```python
from build123d import *

# Parameters (mm, degrees)
F0_R     = 6.35
F1_DEPTH = 3.175
F2_R     = 6.35
F4_DEPTH = 3.175
F5_COUNT = 4
F6_COUNT = 4


with BuildPart() as f1:
    # F0 (on Top) → F1 (new body)
    with BuildSketch(Plane.XY):
        with BuildLine():
            Line((4.7625, -143.2460284405), (4.7625, -9.1539715595))
            ThreePointArc((4.7625, -9.1539715595), (0, 10.31875), (-4.7625, -9.1539715595))
            Line((-4.7625, -9.1539715595), (-4.7625, -143.2460284405))
            ThreePointArc((-4.7625, -143.2460284405), (0, -162.71875), (4.7625, -143.2460284405))
        make_face()
        with Locations((0, -152.4)):
            Circle(F0_R, mode=Mode.SUBTRACT)
        Circle(F0_R, mode=Mode.SUBTRACT)
    extrude(amount=F1_DEPTH)

    # F2
    f2_edges = [f1.edges().sort_by_distance(p)[0] for p in [
        (4.7625, -9.153972, 1.5875),
        (-4.7625, -9.153972, 1.5875),
        (-4.7625, -143.246028, 1.5875),
        (4.7625, -143.246028, 1.5875),
    ]]
    fillet(f2_edges, radius=F2_R)

    # F3 (on face) → F4 (cut, through all)
    with BuildSketch(Plane.XY.offset(3.175)):
        with BuildLine():
            ThreePointArc((-5.8666350314, -154.8300397955), (-6.35, -152.4), (-5.8666350314, -149.9699602045))
            Line((-5.8666350314, -149.9699602045), (-6.5999644104, -149.66620523))
            ThreePointArc((-6.5999644104, -149.66620523), (-7.14375, -152.4), (-6.5999644104, -155.13379477))
            Line((-6.5999644104, -155.13379477), (-5.8666350314, -154.8300397955))
        make_face()
        with BuildLine():
            ThreePointArc((-5.8666350314, -2.4300397955), (-6.35, 0), (-5.8666350314, 2.4300397955))
            Line((-5.8666350314, 2.4300397955), (-6.5999644104, 2.73379477))
            ThreePointArc((-6.5999644104, 2.73379477), (-7.14375, 0), (-6.5999644104, -2.73379477))
            Line((-6.5999644104, -2.73379477), (-5.8666350314, -2.4300397955))
        make_face()
    f4 = extrude(amount=-F4_DEPTH, mode=Mode.SUBTRACT)

    # F5: F4 ×4 about axis
    f5_axis = Axis((0, -152.4, 3.175), (0, 0, 1))
    for i in range(1, F5_COUNT):
        add(f4.solids().sort_by_distance((-6.2333, -154.981917, 1.5875))[0].rotate(f5_axis, i * 360 / F5_COUNT), mode=Mode.SUBTRACT)

    # F6: F4 ×4 about axis
    f6_axis = Axis((0, 0, 3.175), (0, 0, 1))
    for i in range(1, F6_COUNT):
        add(f4.solids().sort_by_distance((-6.2333, 2.581917, 1.5875))[0].rotate(f6_axis, i * 360 / F6_COUNT), mode=Mode.SUBTRACT)


solid = f1.part
```
The listing builds one solid part. Answer for the finished solid, in the listing's coordinates (mm). A direction names the side the tool comes from. Coordinates: 2 decimals unless noted, no trailing zeros. Write each loop counter-clockwise with the first axis right and the second up, starting at its lowest first coordinate (ties: lowest second). Pieces come first, ordered by that corner, then holes. Notation, with made-up numbers: (11.25, 89) - (44.25, 89) arc R29 ccw to (44.25, 113) - close; hole circle Ø11 at (-2.75, 72.5). An arc over 180 degrees is marked (long way). Return JSON: item names as keys, results as strings. Group by question number.
1. A cutting plane is placed at B-B, the plane x = 0. Determine the outline of the cut face in (y, z) (3 decimals), plus the area to 3 significant figures.
2. A cutting plane is placed at A-A, the plane y = -152.4. Determine the outline of the cut face in (x, z) (3 decimals), plus the area to 3 significant figures.
3. Straight lines are drawn through the part: L1, parallel to X at y = -152.5, z = 2.6; L2, parallel to Y at x = 0.25, z = 2.15; L3, parallel to Y at x = 3, z = 1.6. For each, find the intervals that lie inside material, in ascending order.
4. Determine the mould class of faces 4 (the flat face through (0, -75, 3.175)), 5 (the cylindrical face through (-4.47, 4.51, 1.57)) for opening direction Y: released by +Y, released by -Y, zero draft, split by the parting line, or undercut.
5. Which of the six approach directions +Z, -Z, +X, -X, +Y, -Y give full straight-line access (tool end or side, diameter ignored) to faces 1 (the flat face through (4.762, -77, 2)), 2 (the cylindrical face through (-5.33, -9.8, 1.61)), 3 (the cylindrical face through (-0.039, -7.144, 1.61))?
6. A cutting plane is placed at D-D, the plane y = -16.5. Determine the outline of the cut face in (x, z) (1 decimal).
7. A cutting plane is placed at C-C, the plane z = 1.45. Give the number of separate pieces and of enclosed holes in the cut face, plus the area to 3 significant figures.
8. Given pin 1 (1.5 mm diameter, centred on y = -98.5, z = 1.5, fed in from -X), flat-ended and moving along its own axis, determine where the tip first touches the part or whether it passes through.
Ans:
{
 "1": {"outline": "(-162.719, 0) - (-159.544, 0) - (-159.544, 3.175) - (-162.719, 3.175) - close; (-145.256, 0) - (-7.144, 0) - (-7.144, 3.175) - (-145.256, 3.175) - close; (7.144, 0) - (10.319, 0) - (10.319, 3.175) - (7.144, 3.175) - close", "area": "459 mm²"},
 "2": {"outline": "(-10.319, 0) - (-7.144, 0) - (-7.144, 3.175) - (-10.319, 3.175) - close; (7.144, 0) - (10.319, 0) - (10.319, 3.175) - (7.144, 3.175) - close", "area": "20.2 mm²"},
 "3": {"L1": "-10.32 to -7.14, 7.14 to 10.32", "L2": "-162.72 to -159.54, -145.26 to -7.14, 7.14 to 10.32", "L3": "-162.27 to -158, -146.8 to -5.6, 5.6 to 9.87"},
 "4": {"face 4": "zero draft", "face 5": "undercut"},
 "5": {"face 1": "+Z, -Z, +X", "face 2": "+Z, -Z, -X", "face 3": "+Z, -Z"},
 "6": {"outline": "(-4.8, 0) - (4.8, 0) - (4.8, 3.2) - (-4.8, 3.2) - close"},
 "7": {"separate pieces": "1", "enclosed holes": "2", "area": "1,650 mm²"},
 "8": {"pin 1": "x = -4.76"}
}
